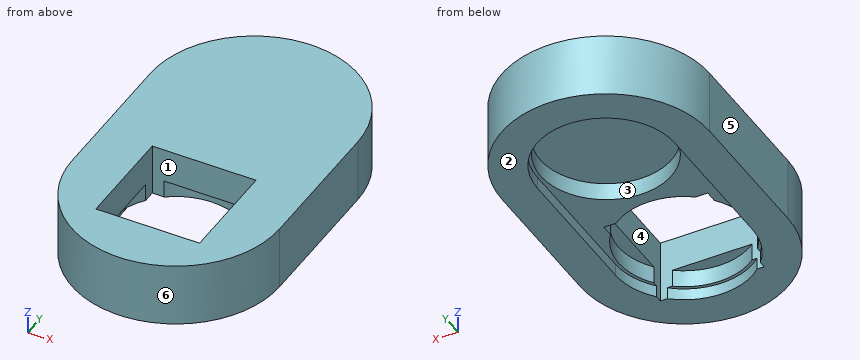
Autodesk Fusion 360 part; units mm, degrees
sketch "Boceto1" plane through (0, 0, 0) normal (0, 0, 1) x (1, 0, 0)
  circle A0 centre (0, 9) radius 13
  circle A1 centre (0, -9) radius 13
  line L0 (-13, -9) -> (-13, 9)
  line L1 (13, -9) -> (13, 9)
extrude "Extruir1" add sketch "Boceto1" along normal blind 8
sketch "Boceto2" plane through (0, 0, 0) normal (0, 0, 1) x (1, 0, 0)
  circle A0 centre (0, 9) radius 8.6
  circle A1 centre (0, -9) radius 8.6
  line L0 (-8.6, -9) -> (-8.6, 9)
  line L1 (8.6, -9) -> (8.6, 9)
extrude "Extruir2" cut sketch "Boceto2" along normal blind 1.5
sketch "Boceto3" plane through (0, 0, 0) normal (0, 0, 1) x (1, 0, 0)
  circle A0 centre (0, 9) radius 8.2
  circle A1 centre (0, -9) radius 8.2
extrude "Extruir3" cut sketch "Boceto3" along normal blind 3.7
sketch "Boceto4" plane through (0, 0, 0) normal (0, 0, 1) x (1, 0, 0)
  line L0 (-6.5, -15.5) -> (6.5, -15.5)
  line L1 (6.5, -15.5) -> (6.5, -2.5)
  line L2 (6.5, -2.5) -> (-6.5, -2.5)
  line L3 (-6.5, -2.5) -> (-6.5, -15.5)
extrude "Extruir4" cut sketch "Boceto4" along normal blind 8
The model under review builds one solid part; all positions refer to its coordinate system, in mm. Face numbers are marked on the shaded views. A direction names the side the tool comes from. Round coordinates to 2 decimals unless told otherwise and drop trailing zeros. Order: outer loops, then holes, each group sorted by start corner. A loop starts at its lowest first (then second) coordinate and runs counter-clockwise, first axis right, second up. Notation, with made-up numbers: (-20.5, 45.5) -> (37.5, 45.5) arc R25 ccw to (37.5, 69.5) -> close; hole circle Ø3 at (-38, -13). An arc over 180 degrees is marked (long way). One line per item, written item: value. Start each with the question number.
Q1. Take a section at B-B (z = 7.25). Write out the cut boundary in (x, y), and give its area (3 significant figures).
Q2. Take a section at D-D (y = 8). Write out the cut boundary in (x, z).
Q3. Mouldability with a two-part tool opening along Y and no side actions: class the marked faces 4, 5 and 6 as released by +Y, released by -Y, zero draft, split by the parting line, or undercut.
Q4. Take a section at C-C (z = 3.25). Write out the cut boundary in (x, y).
Q5. Take a section at A-A (x = 0). Write out the cut boundary in (y, z).
Q6. Clearance check with flat-ended pins moving along their axes: pin 1 Ø1 at (x, z) = (1.5, 4.5) entering from -Y; pin 2 Ø8 at (x, y) = (-3, 5.5) entering from -Z; pin 3 Ø2 at (y, z) = (10.5, 1) entering from +X. State where each tip first meets the part, or that it passes through.
Q7. Machinability: for the marked faces 1, 2 and 3, which of the approach directions +Z, -Z, +X, -X, +Y, -Y give a long, thin tool a straight path to every point of the face, cutting with its end or side? Answer none if there is none.
Q8. Wall thickness on line 1 (Y direction, x = 0, z = 3.15); line 2 (X direction, y = -5.5, z = 6); line 3 (X direction, y = 9, z = 2.7): over which ranges is each line inside the solid? List them lowest first.
Reported:
1. outline: (-13, -9) arc R13 ccw to (13, -9) -> (13, 9) arc R13 ccw to (-13, 9) -> close; hole (-6.5, -15.5) -> (6.5, -15.5) -> (6.5, -2.5) -> (-6.5, -2.5) -> close
1. area: 830 mm2
2. outline: (-13, 0) -> (-8.6, 0) -> (-8.6, 1.5) -> (-8.14, 1.5) -> (-8.14, 3.7) -> (8.14, 3.7) -> (8.14, 1.5) -> (8.6, 1.5) -> (8.6, 0) -> (13, 0) -> (13, 8) -> (-13, 8) -> close
3. face 4: undercut
3. face 5: zero draft
3. face 6: released by -Y
4. outline: (-13, -9) arc R13 ccw to (13, -9) -> (13, 9) arc R13 ccw to (-13, 9) -> close; hole circle Ø16.4 at (0, 9); hole (-6.5, -15.5) -> (-5, -15.5) arc R8.2 ccw to (5, -15.5) -> (6.5, -15.5) -> (6.5, -14) arc R8.2 ccw to (6.5, -4) -> (6.5, -2.5) -> (5, -2.5) arc R8.2 ccw to (-5, -2.5) -> (-6.5, -2.5) -> (-6.5, -4) arc R8.2 ccw to (-6.5, -14) -> close
5. outline: (-22, 0) -> (-17.6, 0) -> (-17.6, 1.5) -> (-17.2, 1.5) -> (-17.2, 3.7) -> (-15.5, 3.7) -> (-15.5, 8) -> (-22, 8) -> close; (-2.5, 3.7) -> (-0.8, 3.7) -> (-0.8, 1.5) -> (0.8, 1.5) -> (0.8, 3.7) -> (17.2, 3.7) -> (17.2, 1.5) -> (17.6, 1.5) -> (17.6, 0) -> (22, 0) -> (22, 8) -> (-2.5, 8) -> close
6. pin 1: stops at y = -21.96
6. pin 2: stops at z = 1.5
6. pin 3: stops at x = 12.99
7. face 1: +Z, -Z
7. face 2: -Z, +X, -X, +Y, -Y
7. face 3: -Z
8. line 1: y = -22 to -17.2, -0.8 to 0.8, 17.2 to 22
8. line 2: x = -13 to -6.5, 6.5 to 13
8. line 3: x = -13 to -8.2, 8.2 to 13
